For this review, take the finished solid that the model builds, in its own axes (mm). A direction names the side the tool comes from. Give positions to 0.01 mm unless a question says otherwise; leave off trailing zeros. Order: outer loops, then holes, each group sorted by start corner. A loop starts at its lowest first (then second) coordinate and runs counter-clockwise, first axis right, second up.
Item 1: Consider section B-B (z = 0.2). Give the boundary of the cut face in (x, y).
Item 2: The part is to be moulded in two halves that separate along Y. For faces 4 (the flat face through (-4.83, -13.3, 0.64)), 5 (the flat face through (-8, 12, 0)), 6 (the cylindrical face through (5.04, -10.18, 0.64)), 7 (the cylindrical face through (6.529, -12.524, 0.641)), say which applies: released by +Y, released by -Y, zero draft, split by the parting line, or undercut.
Item 3: For P1, Ø6, axis at x = -10, y = 1.5, coming from the +Z side, flat-tipped, find the tip position at first contact; note if it passes through.
Item 4: Machinability: for faces 1 (the flat face through (4.83, -13.3, 0.64)), 2 (the flat face through (-7.93, -10.65, 0.64)), 3 (the flat face through (-8, 12, 1.3)), which of the approach directions +Z, -Z, +X, -X, +Y, -Y give a long, thin tool a straight path to every point of the face, cutting with its end or side? Answer none if there is none.
Item 5: Consider section D-D (x = 0). Give the boundary of the cut face in (y, z), plus the area to 3 significant figures.
Item 6: For probe 1 along X at (y, z) = (-11.6, 0.7); probe 2 along Y at (x, z) = (5.5, 0.75); probe 3 along Y at (x, z) = (-13, 0.95), list the stretches that pass through material, from the lowest coordinate up.
Item 7: Consider section A-A (y = 0.7). Give the boundary of the cut face in (x, z).
Item 8: Consider section C-C (y = -11.6). Give the boundary of the cut face in (x, z), plus the area to 3 significant figures.
Autodesk Inventor part; units mm, degrees
ref_plane "WorkPlane1" through (0, 0, 0) normal (0, 0, 1) x (1, 0, 0)
ref_plane "Work Plane2" through (0, 0, -1.3) normal (0, 0, 1) x (1, 0, 0)
ref_plane "WorkPlane2" through (0, 0, 1) normal (0, 0, 1) x (1, 0, 0)
ref_plane "WorkPlane1" through (0, 0, 0) normal (0, 0, 1) x (1, 0, 0)
ref_plane "Work Plane2" through (0, 0, -1.3) normal (0, 0, 1) x (1, 0, 0)
ref_plane "WorkPlane2" through (0, 0, 1) normal (0, 0, 1) x (1, 0, 0)
sketch "Szkic1" plane through (0, 0, 0) normal (0, 0, 1) x (1, 0, 0)
  point P0 (0, 0)
sketch "Szkic2" plane through (0, 0, 0) normal (0, 0, 1) x (1, 0, 0)
  line L0 (5.2, -14.3785) -> (4.4442, -12.1869)
  arc A0 (7.1776, -10.1251) -> (4.4442, -12.1869) centre (6.1458, -11.6) ccw
  line L1 (7.1776, -10.1251) -> (8.7079, -11.1955)
  arc A1 (8.7079, -11.1955) -> (-8.7079, -11.1955) centre (0, 0) ccw
  line L2 (-7.1776, -10.1251) -> (-8.7079, -11.1955)
  arc A2 (-4.4442, -12.1869) -> (-7.1776, -10.1251) centre (-6.1458, -11.6) ccw
  line L3 (-5.2, -14.3785) -> (-4.4442, -12.1869)
  arc A3 (5.2, -14.3785) -> (-5.2, -14.3785) centre (0, 0.7) ccw
  line L4 (0, 0.7) -> (-5.2, -14.3785) construction
  line L5 (0, 0.7) -> (5.2, -14.3785) construction
  dimension "d2" = 15.95
  dimension "d4" = 0
  dimension "d6" = 14.1833
  dimension "d8" = 0.7
  dimension "d10" = 5.2
  dimension "d12" = 5.2
  dimension "d14" = 1.8
  dimension "d16" = 1.8
  dimension "d18" = 13.75
  dimension "d20" = 13.75
  dimension "d22" = 36
  dimension "d24" = 36
extrude "Wyciągnięcie proste1" add sketch "Szkic2" along normal blind 1.3
sketch "Szkic3" plane through (0, 0, 1.3) normal (0, 0, 1) x (1, 0, 0)
  arc A0 (-4.4442, -12.1869) -> (-7.1776, -10.1251) centre (-6.1458, -11.6) ccw
hole "Otwór1" at (-6.1458, -11.6, 1.3) direction (0, 0, -1) diameter 2 end through all
sketch "Szkic4" plane through (0, 0, 1.3) normal (0, 0, 1) x (1, 0, 0)
  arc A0 (7.1776, -10.1251) -> (4.4442, -12.1869) centre (6.1458, -11.6) ccw
hole "Otwór2" at (6.1458, -11.6, 1.3) direction (0, 0, -1) diameter 2 end through all
equation "\"d2\" = 0.5 * Diam2"
equation "\"d6\" = 0.5 * msp_dd1"
equation "\"d8\" = -0.5 * msp_dd1 + 0.5 * Diam2 - 0.222222 * ParA"
equation "\"d10\" = 2.6 * Diam5"
equation "\"d12\" = 2.6 * Diam5"
equation "\"d14\" = 0.9 * Diam5"
equation "\"d16\" = 0.9 * Diam5"
equation "\"d18\" = 1.3 * Diam5 + 0.5 * Diam2 - ParA"
equation "\"d20\" = 1.3 * Diam5 + 0.5 * Diam2 - ParA"
equation "\"d25\" = ParS"
equation "\"d29\" = Diam5"
equation "\"d36\" = Diam5"
equation "\"Diam5\" = 2"
equation "\"ParA\" = 4.8"
equation "\"ParS\" = 1.3"
equation "\"Diam2\" = 31.9"
equation "\"msp_dd1\" = -b + Diam2 - 0.111111 * ParA"
equation "\"msp_pom\" = 0.5 * Diam2 - b"
equation "\"TEMPLATE\" = 1.2345"
properties part number "ANSI B 27.7M - 3BMI-30" material "Stal, miękka"
Resolved:
1. outline: (-8.71, -11.2) arc R14.18 cw (long way) to (8.71, -11.2) - (7.18, -10.13) arc R1.8 ccw to (4.44, -12.19) - (5.2, -14.38) arc R15.95 ccw (long way) to (-5.2, -14.38) - (-4.44, -12.19) arc R1.8 ccw to (-7.18, -10.13) - close; hole circle Ø2 at (-6.15, -11.6); hole circle Ø2 at (6.15, -11.6)
2. face 4: released by -Y
2. face 5: zero draft
2. face 6: undercut
2. face 7: undercut
3. P1: passes through
4. face 1: +Z, -Z, -Y
4. face 2: +Z, -Z
4. face 3: +Z, +X, -X, +Y, -Y
5. outline: (14.18, 0) - (16.65, 0) - (16.65, 1.3) - (14.18, 1.3) - close
5. area: 3.21 mm2
6. probe 1: x = -10.15 to -7.15, -5.15 to -4.35, 4.35 to 5.15, 7.15 to 10.15
6. probe 2: y = -14.27 to -12.36, -10.84 to -9.92, 13.07 to 15.67
6. probe 3: y = -8.54 to -5.67, 5.67 to 9.94
7. outline: (-15.95, 0) - (-14.17, 0) - (-14.17, 1.3) - (-15.95, 1.3) - close; (14.17, 0) - (15.95, 0) - (15.95, 1.3) - (14.17, 1.3) - close
8. outline: (-10.15, 0) - (-7.15, 0) - (-7.15, 1.3) - (-10.15, 1.3) - close; (-5.15, 0) - (-4.35, 0) - (-4.35, 1.3) - (-5.15, 1.3) - close; (4.35, 0) - (5.15, 0) - (5.15, 1.3) - (4.35, 1.3) - close; (7.15, 0) - (10.15, 0) - (10.15, 1.3) - (7.15, 1.3) - close
8. area: 9.90 mm2
